Verification items for the finished model (mm, model axes). A direction names the side the tool comes from. Give positions to 0.01 mm unless a question says otherwise; leave off trailing zeros. Write each loop counter-clockwise with the first axis right and the second up, starting at its lowest first coordinate (ties: lowest second). Pieces come first, ordered by that corner, then holes. Notation, with made-up numbers: (34.5, 53) -> (63.5, 53) arc R16 cw to (63.5, 64) -> close; hole circle Ø2 at (54, -31). An arc over 180 degrees is marked (long way). Write item = value, one per line.
from build123d import *

# Parameters (mm, degrees)
SKETCH_4_R          = 17
EXTRUDE_2_DEPTH     = 2
SKETCH_5_R          = 15
EXTRUDE_3_DEPTH     = 4
CUT_EXTRUDE_1_DEPTH = 2.6
SKETCH_7_R          = 3.55
CUT_EXTRUDE_2_DEPTH = 1.4
SKETCH_8_R          = 2
CUT_EXTRUDE_3_DEPTH = 25.280856657
SKETCH_9_R          = 5.5
CUT_EXTRUDE_4_DEPTH = 1
SKETCH_11_R         = 1.65
CUT_EXTRUDE_5_DEPTH = 25.309668858
SKETCH_13_R         = 1.5
CUT_EXTRUDE_6_DEPTH = 25.779023387


with BuildPart() as part:
    # 草图4 → 凸台-拉伸2 (new body)
    with BuildSketch(Plane(origin=(0, 0, 0), x_dir=(0, 0, -1), z_dir=(1, 0, 0))):
        Circle(SKETCH_4_R)
    extrude(amount=EXTRUDE_2_DEPTH)

    # 草图5 → 凸台-拉伸3 (add)
    with BuildSketch(Plane(origin=(2, 0, 0), x_dir=(0, 0, -1), z_dir=(1, 0, 0))):
        Circle(SKETCH_5_R)
    extrude(amount=EXTRUDE_3_DEPTH)

    # 草图6 → 切除-拉伸1 (cut)
    with BuildSketch(Plane.ZY):
        with BuildLine():
            Line((-3.031088913, 12.75), (-12.557368355, -3.75))
            ThreePointArc((-12.557368355, -3.75), (-12.557368355, -7.25), (-9.526279442, -9))
            Line((-9.526279442, -9), (9.526279442, -9))
            ThreePointArc((9.526279442, -9), (12.557368355, -7.25), (12.557368355, -3.75))
            Line((12.557368355, -3.75), (3.031088913, 12.75))
            ThreePointArc((3.031088913, 12.75), (0, 14.5), (-3.031088913, 12.75))
        make_face()
    extrude(amount=-CUT_EXTRUDE_1_DEPTH, mode=Mode.SUBTRACT)

    # 草图7 → 切除-拉伸2 (cut)
    with BuildSketch(Plane.ZY.offset(-2.6)):
        with Locations((0, 10.2)):
            Circle(SKETCH_7_R)
        with Locations((8.833459119, -5.1)):
            Circle(SKETCH_7_R)
        with Locations((-8.833459119, -5.1)):
            Circle(SKETCH_7_R)
    extrude(amount=-CUT_EXTRUDE_2_DEPTH, mode=Mode.SUBTRACT)

    # 草图8 → 切除-拉伸3 (cut, through all)
    with BuildSketch(Plane.ZY.offset(-2.6)):
        with Locations((0, 10.2)):
            Circle(SKETCH_8_R)
        with Locations((8.833459119, -5.1)):
            Circle(SKETCH_8_R)
        with Locations((-8.833459119, -5.1)):
            Circle(SKETCH_8_R)
    extrude(amount=-CUT_EXTRUDE_3_DEPTH, mode=Mode.SUBTRACT)

    # 草图9 → 切除-拉伸4 (cut)
    with BuildSketch(Plane.ZY.offset(-2.6)):
        Circle(SKETCH_9_R)
    extrude(amount=-CUT_EXTRUDE_4_DEPTH, mode=Mode.SUBTRACT)

    # 草图11 → 切除-拉伸5 (cut, through all)
    with BuildSketch(Plane.ZY.offset(-3.6)):
        Circle(SKETCH_11_R)
    extrude(amount=-CUT_EXTRUDE_5_DEPTH, mode=Mode.SUBTRACT)

    # 草图13 → 切除-拉伸6 (cut, through all)
    with BuildSketch(Plane(origin=(6, 0, 0), x_dir=(0, 0, -1), z_dir=(1, 0, 0))):
        with Locations((-8.833459119, 5.1)):
            Circle(SKETCH_13_R)
        with Locations((8.833459119, 5.1)):
            Circle(SKETCH_13_R)
        with Locations((0, -10.2)):
            Circle(SKETCH_13_R)
    extrude(amount=-CUT_EXTRUDE_6_DEPTH, mode=Mode.SUBTRACT)


solid = part.part
Item 1: Sectioned sample at B-B on z = 0. Give the number of separate pieces and of enclosed holes in the cut face, then the cut area to 3 significant figures.
Response values:
separate_pieces = 4
enclosed_holes = 0
area = 72.8 mm^2
Item 2: Mould release check, pull along Z, two halves, no side actions. Record for faces 1 (the flat face through (0, 8, -7)), 2 (the cylindrical face through (3.972, 0.66, 14.985)), 3 (the cylindrical face through (3.042, -11.664, 0.325)): +Z half, -Z half, draft (parallel to the pull), parting line (faces both ways), or undercut.
Response values:
face_1 = draft
face_2 = parting line
face_3 = undercut
Item 3: Go/stop test with flat-tipped pins: P1, Ø6.5, axis at y = -5.1, z = -8.83, coming from the +X side; P2, Ø5.5, axis at y = -5.1, z = 8.83, coming from the -X side; P3, Ø3, axis at x = 1, z = -7, coming from the +Y side; P4, Ø3, axis at x = 4.5, z = -3, coming from the -Y side. Record where each tip stops, or that it passes through.
Response values:
P1 = 6
P2 = 4
P3 = 16.09
P4 = -14.92
Item 4: Sectioned sample at A-A on x = 5. Record the cut outline in (y, z), then the cut area to 3 significant figures.
Response values:
outline = circle Ø30 at (0, 0); hole circle Ø3 at (-10.2, 0); hole circle Ø4 at (-5.1, -8.83); hole circle Ø4 at (-5.1, 8.83); hole circle Ø3.3 at (0, 0); hole circle Ø3 at (5.1, -8.83); hole circle Ø3 at (5.1, 8.83); hole circle Ø4 at (10.2, 0)
area = 639 mm^2
Item 5: Sectioned sample at C-C on y = 11. Record the cut outline in (x, z), then the cut area to 3 significant figures.
Response values:
outline = (0, -12.96) -> (2, -12.96) -> (2, -10.2) -> (6, -10.2) -> (6, -1.83) -> (4, -1.83) -> (4, -3.46) -> (2.6, -3.46) -> (2.6, -4.04) -> (0, -4.04) -> close; (0, 4.04) -> (2.6, 4.04) -> (2.6, 3.46) -> (4, 3.46) -> (4, 1.83) -> (6, 1.83) -> (6, 10.2) -> (2, 10.2) -> (2, 12.96) -> (0, 12.96) -> close
area = 95.4 mm^2
Item 6: Material ranges on line 1 (Y direction, x = 3.4, z = 0); line 2 (X direction, y = -5, z = 1); line 3 (Y direction, x = 2.35, z = 12), recorded low to high.
Response values:
line_1 = -15 to -11.7, -8.7 to -5.5, 5.5 to 6.65, 13.75 to 15
line_2 = 3.6 to 6
line_3 = -9 to -7.98, -2.78 to 9
Item 7: Set-up check for faces 4 (the flat face through (2, -14, -6)), 5 (the cylindrical face through (1.282, -7.294, 12.531)), 6 (the cylindrical face through (4.986, -4.499, -6.926)): record each of +Z, -Z, +X, -X, +Y, -Y from which the full face is reachable in a straight line by a thin tool's end or side.
Response values:
face_4 = +X
face_5 = -X
face_6 = +X, -X
